Answer from the drawing. Dimensions are ordinates in mm from the lowest x, y and z of the part. A direction names the side the tool comes from. Coordinates: 2 decimals unless noted, no trailing zeros. Order: outer loops, then holes, each group sorted by start corner. A loop starts at its lowest first (then second) coordinate and runs counter-clockwise, first axis right, second up.
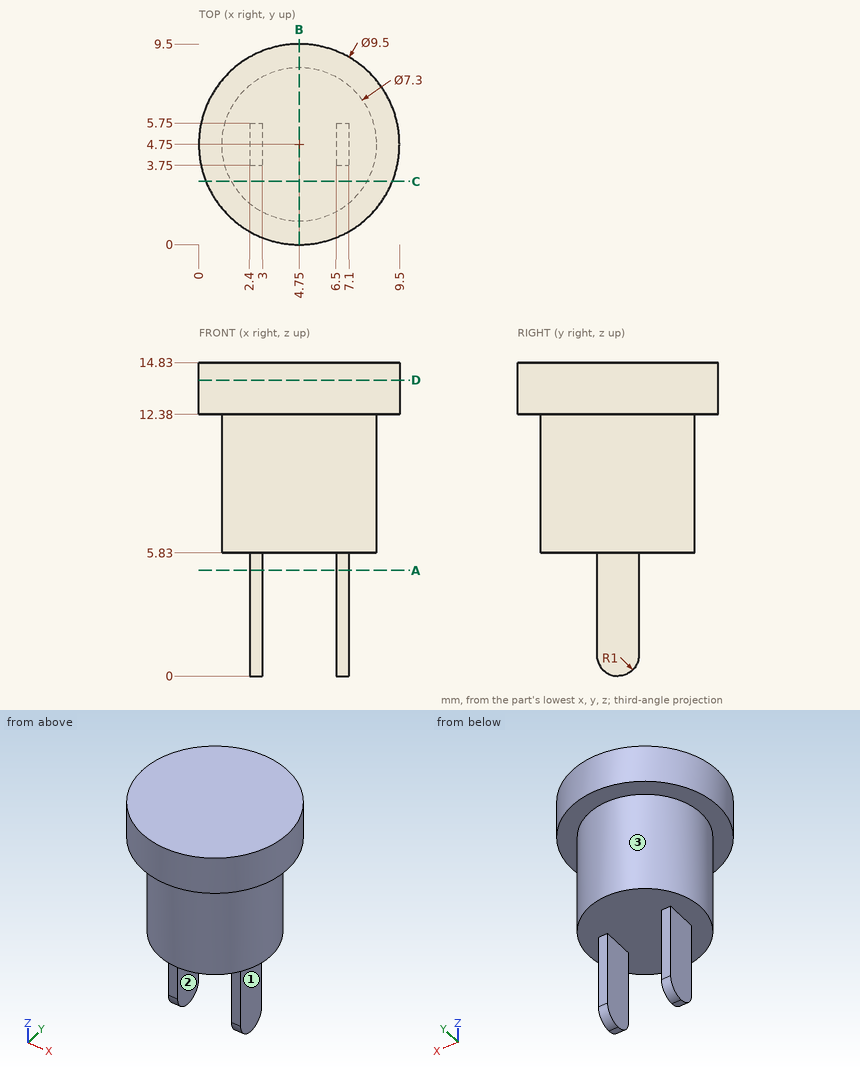
1. For the marked faces 1, 2 and 3, determine the directions among +Z, -Z, +X, -X, +Y, -Y from which every point of the face is accessible in a straight line to the end or side of a thin tool.
2. The part is cut by section D-D (z = 14). Determine the outline of the cut face in (x, y), plus the area to 3 significant figures.
3. Consider probe 1 along X at (y, z) = (4.5, 4.25); probe 2 along Z at (x, y) = (6.75, 3.5); probe 3 along Y at (x, z) = (4.75, 9). Determine where each line is inside the solid, lowest interval first.
4. The part is cut by section B-B (x = 4.75). Determine the outline of the cut face in (y, z).
5. The part is cut by section C-C (y = 3). Determine the outline of the cut face in (x, z), plus the area to 3 significant figures.
6. The part is cut by section A-A (z = 5). Determine the outline of the cut face in (x, y), plus the area to 3 significant figures.
7. Flat-ended cylindrical pins translate along their axes: pin 1 (3 mm diameter, centred on y = 3, z = 3.5, fed in from +X); pin 2 (1.6 mm diameter, centred on y = 5, z = 2, fed in from -X); pin 3 (5 mm diameter, centred on x = 2, z = 3, fed in from -Y). Find the tip coordinate at first contact, or state that the pin passes through.
Worked out:
1. face 1: -Z, +X, +Y, -Y
1. face 2: -Z, +Y, -Y
1. face 3: -Z
2. outline: circle Ø9.5 at (4.75, 4.75)
2. area: 70.9 mm2
3. probe 1: x = 2.4 to 3, 6.5 to 7.1
3. probe 2: z = 5.83 to 14.83
3. probe 3: y = 1.1 to 8.4
4. outline: (0, 12.38) - (1.1, 12.38) - (1.1, 5.83) - (8.4, 5.83) - (8.4, 12.38) - (9.5, 12.38) - (9.5, 14.83) - (0, 14.83) - close
5. outline: (0.33, 12.38) - (1.55, 12.38) - (1.55, 5.83) - (7.95, 5.83) - (7.95, 12.38) - (9.17, 12.38) - (9.17, 14.83) - (0.33, 14.83) - close
5. area: 63.6 mm2
6. outline: (2.4, 3.75) - (3, 3.75) - (3, 5.75) - (2.4, 5.75) - close; (6.5, 3.75) - (7.1, 3.75) - (7.1, 5.75) - (6.5, 5.75) - close
6. area: 2.40 mm2
7. pin 1: stops at x = 7.1
7. pin 2: stops at x = 2.4
7. pin 3: stops at y = 3.75
